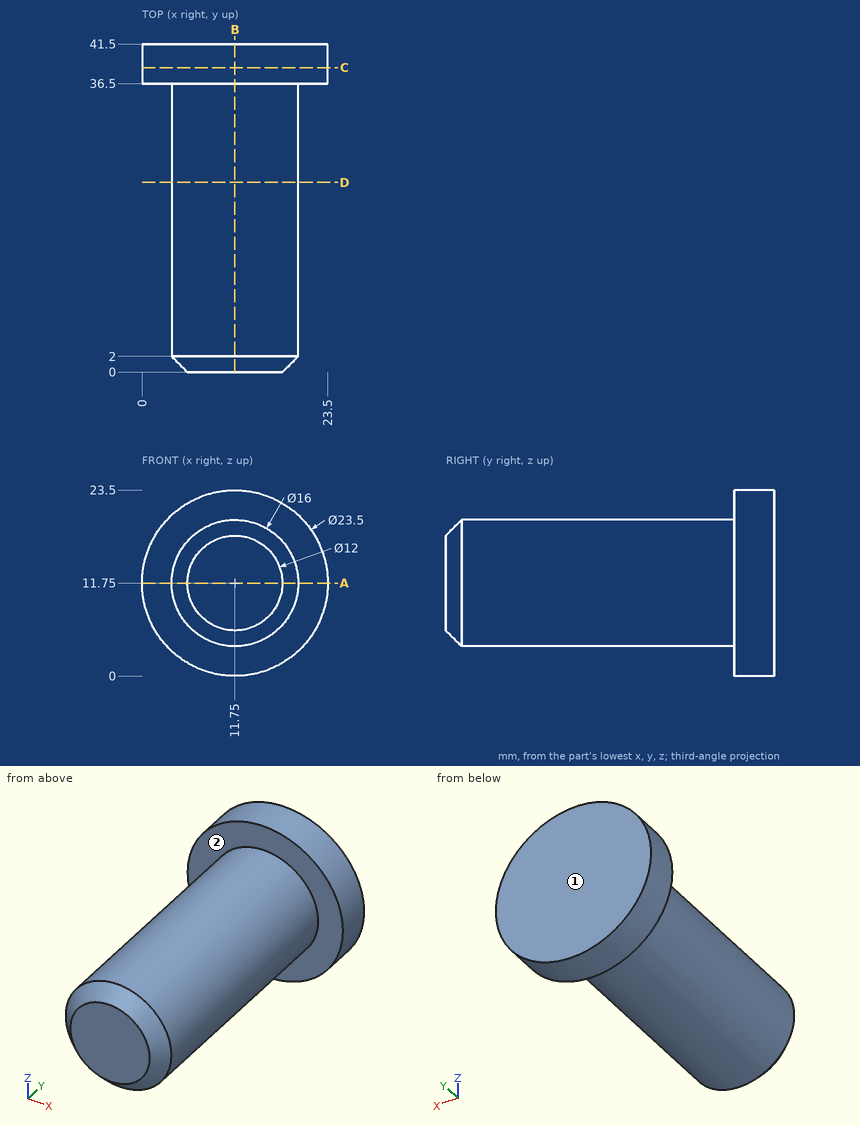
Drawing for the job (mm, zero at the part's lowest x, y, z). A direction names the side the tool comes from. Coordinates: 2 decimals unless noted, no trailing zeros. Order: outer loops, then holes, each group sorted by start corner. A loop starts at its lowest first (then second) coordinate and runs counter-clockwise, first axis right, second up. Notation, with made-up numbers: (32, 24.25) -> (52, 24.25) arc R36 cw to (52, 61.25) -> close; hole circle Ø4 at (83.25, 81). An arc over 180 degrees is marked (long way). One line per item, written item: value.
(1) Slice it at B-B, the plane x = 11.75. List the corners of the cut face in (y, z).
Checked values:
outline: (0, 5.75) -> (2, 3.75) -> (36.5, 3.75) -> (36.5, 0) -> (41.5, 0) -> (41.5, 23.5) -> (36.5, 23.5) -> (36.5, 19.75) -> (2, 19.75) -> (0, 17.75) -> close
(2) Drop flat-ended pins along their axis: pin 1 Ø1 at (x, y) = (14.5, 23) entering from -Z; pin 2 Ø10 at (y, z) = (4.5, 12) entering from -X; pin 3 Ø1.5 at (x, y) = (4, 14.5) entering from -Z. Give the stop position or say it passes through.
Checked values:
pin 1: z = 4.07
pin 2: x = 3.75
pin 3: z = 7.88
(3) Probe line 1 (Y direction, x = 20.5, z = 9); line 2 (X direction, y = 3.5, z = 15.75); line 3 (X direction, y = 37.5, z = 7). List the from-to ranges inside material, lowest first. Write a range as [from, to].
Checked values:
line 1: [36.5, 41.5]
line 2: [4.82, 18.68]
line 3: [1, 22.5]
(4) Tool access for the marked faces 1 and 2: list every direction of +Z, -Z, +X, -X, +Y, -Y with a clear straight run to the whole face (end or side of a thin tool).
Checked values:
face 1: +Z, -Z, +X, -X, +Y
face 2: -Y
(5) Slice it at A-A, the plane z = 11.75. List the corners of the cut face in (x, y), plus the area to 4 significant figures.
Checked values:
outline: (0, 36.5) -> (3.75, 36.5) -> (3.75, 2) -> (5.75, 0) -> (17.75, 0) -> (19.75, 2) -> (19.75, 36.5) -> (23.5, 36.5) -> (23.5, 41.5) -> (0, 41.5) -> close
area: 697.5 mm2
(6) Slice it at C-C, the plane y = 38.5. List the corners of the cut face in (x, z).
Checked values:
outline: circle Ø23.5 at (11.75, 11.75)
(7) Slice it at D-D, the plane y = 24. List the corners of the cut face in (x, z), plus the area to 3 significant figures.
Checked values:
outline: circle Ø16 at (11.75, 11.75)
area: 201 mm2
